For this review, take the finished solid that the model builds, in its own axes (mm). Coordinates: 2 decimals unless noted, no trailing zeros. Loops run counter-clockwise (first coordinate to the right, second up) from the corner with the lowest first, then second, coordinate; pieces in that order, holes last. Notation, with made-up numbers: (56.5, 87.5) -> (115.5, 87.5) arc R25 cw to (115.5, 117.5) -> close; hole circle Ø8 at (79.25, 44.25). An arc over 180 degrees is marked (long way). One line per item, written item: value.
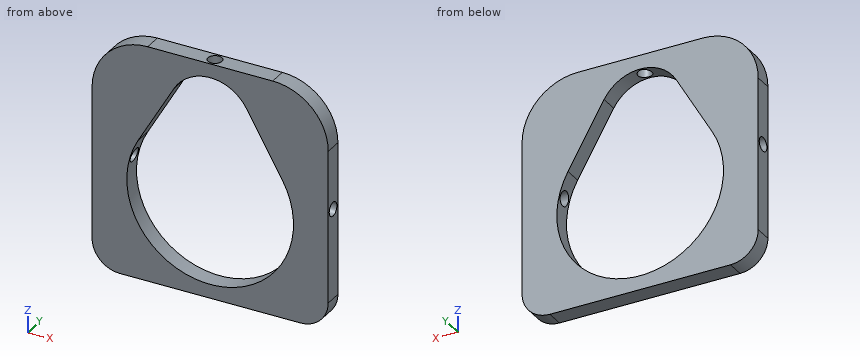
from build123d import *

# Parameters (mm, degrees)
SKETCH1_W           = 85
SKETCH1_H           = 85
BOSS_EXTRUDE1_DEPTH = 6.3
CUT_EXTRUDE1_DEPTH  = 10
CUT_EXTRUDE2_REACH  = 87
SKETCH3_R           = 2.5
SKETCH4_R           = 2.5
CUT_EXTRUDE3_DEPTH  = 86
FILLET1_R           = 20
FILLET2_R           = 10


with BuildPart() as part:
    # Sketch1 → Boss-Extrude1 (new body)
    with BuildSketch(Plane(origin=(0, 0, 0), x_dir=(1, 0, 0), z_dir=(0, 1, 0))):
        with Locations((42.5, 42.5)):
            Rectangle(SKETCH1_W, SKETCH1_H)
    extrude(amount=BOSS_EXTRUDE1_DEPTH)

    # Sketch2 → Cut-Extrude1 (cut)
    with BuildSketch(Plane(origin=(0, 6.3, 0), x_dir=(1, 0, 0), z_dir=(0, 1, 0))):
        with BuildLine():
            Line((16.519237886, 35), (29.509618943, 12.5))
            ThreePointArc((29.509618943, 12.5), (42.5, 5), (55.490381057, 12.5))
            Line((55.490381057, 12.5), (68.480762114, 35))
            ThreePointArc((68.480762114, 35), (42.5, 80), (16.519237886, 35))
        make_face()
    extrude(amount=-CUT_EXTRUDE1_DEPTH, mode=Mode.SUBTRACT)

    # Sketch3 → Cut-Extrude2 (cut, up to next)
    with BuildSketch(Plane.XY, mode=Mode.PRIVATE) as cut_extrude2_sk1:
        with Locations((42.5, 3.15)):
            Circle(SKETCH3_R)
    cut_extrude2_tool1 = extrude(cut_extrude2_sk1.sketch, amount=-CUT_EXTRUDE2_REACH, mode=Mode.PRIVATE) & part.part
    add(cut_extrude2_tool1.solids().sort_by_distance((42.5, 3.15, 0))[0], mode=Mode.SUBTRACT)

    # Sketch4 → Cut-Extrude3 (cut, through all)
    with BuildSketch(Plane.ZY):
        with Locations((-42.5, 3.15)):
            Circle(SKETCH4_R)
    extrude(amount=-CUT_EXTRUDE3_DEPTH, mode=Mode.SUBTRACT)

    # Fillet1
    fillet1_edges = [part.edges().sort_by_distance(p)[0] for p in [
        (85, 3.15, 0),
        (0, 3.15, 0),
    ]]
    fillet(fillet1_edges, radius=FILLET1_R)

    # Fillet2
    fillet2_edges = [part.edges().sort_by_distance(p)[0] for p in [
        (0, 3.15, -85),
        (85, 3.15, -85),
    ]]
    fillet(fillet2_edges, radius=FILLET2_R)


solid = part.part
1. Take a section at B-B, the plane z = -50. Give the boundary of the cut face in (x, y).
Return value:
outline: (0, 0) -> (12.5, 0) -> (12.5, 6.3) -> (0, 6.3) -> close; (72.5, 0) -> (85, 0) -> (85, 6.3) -> (72.5, 6.3) -> close
2. To check wall thickness, follow probe 1 along X at (y, z) = (3, -50); probe 2 along Y at (x, z) = (76, -42.5); probe 3 along X at (y, z) = (0.75, -41). State the ranges of each line that lie inside material, in increasing order. Write a range as from..to.
Return value:
probe 1: x = 0..12.5, 72.5..85
probe 2: y = 0..0.65, 5.65..6.3
probe 3: x = 0..13.88, 71.12..85
3. Take a section at D-D, the plane x = 62.5. Give the boundary of the cut face in (y, z), and give its area (3 significant figures).
Return value:
outline: (0, -85) -> (6.3, -85) -> (6.3, -72.36) -> (0, -72.36) -> close; (0, -24.64) -> (6.3, -24.64) -> (6.3, 0) -> (0, 0) -> close
area: 235 mm2
4. Take a section at A-A, the plane x = 42.5. Give the boundary of the cut face in (y, z), and give its area (3 significant figures).
Return value:
outline: (0, -85) -> (6.3, -85) -> (6.3, -80) -> (0, -80) -> close; (0, -5) -> (0.65, -5) -> (0.65, 0) -> (0, 0) -> close; (5.65, -5) -> (6.3, -5) -> (6.3, 0) -> (5.65, 0) -> close
area: 38.0 mm2
5. Insertion check: pin 1 Ø3 at (x, y) = (42.5, 3.15) entering from +Z. The pin has a flat end and moves straight along its axis. Give the tip position at first contact, or say it passes through.
Return value:
pin 1: stops at z = -79.96
6. Take a section at C-C, the plane y = 3.15. Give the boundary of the cut face in (x, z).
Return value:
outline: (0, -75) arc R10 ccw to (10, -85) -> (75, -85) arc R10 ccw to (85, -75) -> (85, -45) -> (72.08, -45) arc R30 cw (long way) to (12.92, -45) -> (0, -45) -> close; (0, -40) -> (14.22, -40) arc R30 cw to (16.52, -35) -> (29.51, -12.5) arc R15 cw to (40, -5.21) -> (40, 0) -> (20, 0) arc R20 ccw to (0, -20) -> close; (45, -5.21) arc R15 cw to (55.49, -12.5) -> (68.48, -35) arc R30 cw to (70.78, -40) -> (85, -40) -> (85, -20) arc R20 ccw to (65, 0) -> (45, 0) -> close
